from build123d import *

# Parameters (mm, degrees)
SKETCH_1_W           = 50
SKETCH_1_H           = 19
EXTRUDE_1_DEPTH      = 1.7
SKETCH_2_W           = 5
SKETCH_2_H           = 8
EXTRUDE_2_DEPTH      = 3
SKETCH_3_W           = 3
SKETCH_3_H           = 3
EXTRUDE_3_DEPTH      = 2
SKETCH_4_W           = 37
SKETCH_4_H           = 1
EXTRUDE_4_DEPTH      = 4
EXTRUDE_4_DEPTH_BACK = 10.7
SKETCH_6_W           = 3
SKETCH_6_H           = 2
EXTRUDE_6_DEPTH      = 1
SKETCH_7_W           = 3
SKETCH_7_H           = 4
EXTRUDE_7_DEPTH      = 2


with BuildPart() as part:
    # Эскиз1 → Бобышка-Вытянуть1 (new body)
    with BuildSketch(Plane(origin=(0, 0, 0), x_dir=(1, 0, 0), z_dir=(0, 1, 0))):
        Rectangle(SKETCH_1_W, SKETCH_1_H)
    extrude(amount=EXTRUDE_1_DEPTH)

    # Эскиз2 → Бобышка-Вытянуть2 (add)
    with BuildSketch(Plane(origin=(0, 1.7, 0), x_dir=(1, 0, 0), z_dir=(0, 1, 0))):
        with Locations((-22.5, 0)):
            Rectangle(SKETCH_2_W, SKETCH_2_H)
    extrude(amount=EXTRUDE_2_DEPTH)

    # Эскиз3 → Бобышка-Вытянуть3 (add)
    with BuildSketch(Plane(origin=(0, 1.7, 0), x_dir=(1, 0, 0), z_dir=(0, 1, 0))):
        with Locations((-21.5, -8)):
            Rectangle(SKETCH_3_W, SKETCH_3_H)
    extrude(amount=EXTRUDE_3_DEPTH)

    # Эскиз4 → Бобышка-Вытянуть4 (add, two sides)
    with BuildSketch(Plane(origin=(0, 1.7, 0), x_dir=(1, 0, 0), z_dir=(0, 1, 0))) as extrude_4_sk:
        with Locations((1.5, 7.5)):
            Rectangle(SKETCH_4_W, SKETCH_4_H)
        with Locations((1.5, -7.5)):
            Rectangle(SKETCH_4_W, SKETCH_4_H)
    extrude(amount=EXTRUDE_4_DEPTH)
    extrude(extrude_4_sk.sketch, amount=-EXTRUDE_4_DEPTH_BACK)

    # Эскиз6 → Бобышка-Вытянуть6 (add)
    with BuildSketch(Plane.XZ):
        with Locations((-23.5, 0)):
            Rectangle(SKETCH_6_W, SKETCH_6_H)
    extrude(amount=EXTRUDE_6_DEPTH)

    # Эскиз7 → Бобышка-Вытянуть7 (add)
    with BuildSketch(Plane(origin=(0, 1.7, 0), x_dir=(1, 0, 0), z_dir=(0, 1, 0))):
        with Locations((24.5, 0)):
            Rectangle(SKETCH_7_W, SKETCH_7_H)
    extrude(amount=EXTRUDE_7_DEPTH)


solid = part.part
Here's how the part is built. I have some questions about the finished solid (model axes, mm). A direction names the side the tool comes from. Coordinates: 2 decimals unless noted, no trailing zeros. Loops run counter-clockwise (first coordinate to the right, second up) from the corner with the lowest first, then second, coordinate; pieces in that order, holes last.
1. I need wall thicknesses on L1, parallel to Z at x = -15.5, y = -4.25; L2, parallel to Z at x = -21, y = 2.5; L3, parallel to Y at x = -21, z = -4.5. Which ranges of each line are inside material? Lowest first, please.
2. For P1, Ø3, axis at x = 1.5, y = 4, coming from the -Z side; P2, Ø2, axis at x = -21, y = 3, coming from the -Z side; P3, Ø0.5, axis at y = -4, z = -7.5, coming from the -X side, each with a flat end and sliding along its axis, tell me the tip position at first contact or that it passes through.
3. Imagine slicing it at B-B, the plane y = -2.75. Please give me the cut outline in (x, z), and give its area (3 significant figures).
4. Imagine slicing it at D-D, the plane x = -21.5. Please give me the cut outline in (y, z).
5. For faces 4 (the flat face through (-17, 3.7, 7.5)), 5 (the flat face through (1, 4, -7)), 6 (the flat face through (24, 3, -2)), 7 (the flat face through (1, -4, 7)), which set-ups out of +Z, -Z, +X, -X, +Y, -Y let a thin tool reach every point of the face, with its end or its side?
6. Imagine slicing it at A-A, the plane y = 2.5. Please give me the cut outline in (x, z).
7. Imagine slicing it at C-C, the plane z = -0.25. Please give me the cut outline in (x, y).
8. If we mould it in two halves opening along X, with no side actions, what happens to faces 1 (the flat face through (1, 4, -8)), 2 (the flat face through (-20, 3, 8)), 3 (the flat face through (25, 1, 0))? For each: pulls with the +X half, pulls with the -X half, needs draft (parallel to the pull), parting line crosses it, or undercut.
Taken from the geometry:
1. L1: z = -8 to -7, 7 to 8
1. L2: z = -4 to 4, 6.5 to 9.5
1. L3: y = 0 to 1.7
2. P1: stops at z = -8
2. P2: stops at z = -4
2. P3: stops at x = -17
3. outline: (-17, -8) - (20, -8) - (20, -7) - (-17, -7) - close; (-17, 7) - (20, 7) - (20, 8) - (-17, 8) - close
3. area: 74.0 mm2
4. outline: (0, -9.5) - (1.7, -9.5) - (1.7, -4) - (4.7, -4) - (4.7, 4) - (1.7, 4) - (1.7, 6.5) - (3.7, 6.5) - (3.7, 9.5) - (0, 9.5) - close
5. face 4: +Z, -Z, +Y
5. face 5: +X, -X, +Y
5. face 6: -Z, +X, +Y
5. face 7: +X, -X, -Y
6. outline: (-25, -4) - (-20, -4) - (-20, 4) - (-25, 4) - close; (-23, 6.5) - (-20, 6.5) - (-20, 9.5) - (-23, 9.5) - close; (-17, -8) - (20, -8) - (20, -7) - (-17, -7) - close; (-17, 7) - (20, 7) - (20, 8) - (-17, 8) - close; (23, -2) - (26, -2) - (26, 2) - (23, 2) - close
7. outline: (-25, -1) - (-22, -1) - (-22, 0) - (25, 0) - (25, 1.7) - (26, 1.7) - (26, 3.7) - (23, 3.7) - (23, 1.7) - (-20, 1.7) - (-20, 4.7) - (-25, 4.7) - close
8. face 1: needs draft
8. face 2: undercut
8. face 3: pulls with the +X half
